from build123d import *

# Parameters (mm, degrees)
CYLINDER1393_R     = 1.7
CYLINDER1393_DEPTH = 8.5
CYLINDER1391_R     = 3.5
CYLINDER1391_DEPTH = 8.5


with BuildPart() as cylinder1393:
    # Cylinder1393 → Cylinder1393 (new body)
    with BuildSketch(Plane(origin=(436, 67, 100), x_dir=(0, 0, -1), z_dir=(1, 0, 0))):
        Circle(CYLINDER1393_R)
    extrude(amount=CYLINDER1393_DEPTH)


with BuildPart() as bucket_right_half_long_spacer:
    # Cylinder1391 → Cylinder1391 (new body)
    with BuildSketch(Plane(origin=(436, 67, 100), x_dir=(0, 0, -1), z_dir=(1, 0, 0))):
        Circle(CYLINDER1391_R)
    extrude(amount=CYLINDER1391_DEPTH)

    # Cut014358: cut Cylinder1393
    add(cylinder1393.part, mode=Mode.SUBTRACT)


with BuildPart() as bucket_right_half_long_spacer_1:
    # Cut014358 placement: moved
    add(bucket_right_half_long_spacer.part.moved(Location((42, 0, 0))))


solid = bucket_right_half_long_spacer_1.part
Work out the finished part from the listing and answer in its coordinate system (mm). Coordinates: 2 decimals unless noted, no trailing zeros. Loops run counter-clockwise (first coordinate to the right, second up) from the corner with the lowest first, then second, coordinate; pieces in that order, holes last. Notation, with made-up numbers: M 70.25,-16 L 98.25,-16 A22 cw 98.25,7 Z; hole C 47,30 d5. An arc over 180 degrees is marked long. Answer in a Markdown table with one row per item. Add a question column.
1. The mould has two halves that part along Z. Classify faces 1 (the flat face through (478, 68, 98)), 2 (the cylindrical face through (482.19, 67.07, 101.7)), 3 (the cylindrical face through (482.19, 65.659, 96.767)): pulls with the +Z half, pulls with the -Z half, needs draft (parallel to the pull), parting line crosses it, or undercut.
2. Find section B-B, the plane y = 67. Write down the section's boundary in (x, z), then the cut area to 3 significant figures.
3. Consider L1, parallel to Y at x = 482.75, z = 100; L2, parallel to Y at x = 480.25, z = 98.75; L3, parallel to Z at x = 479, y = 68.25. Determine where each line is inside the solid, lowest interval first.
4. Flat-ended cylindrical pins translate along their axes: P1, Ø2, axis at x = 482.5, y = 68, coming from the -Z side; P2, Ø3, axis at y = 67, z = 100, coming from the -X side. Find the tip coordinate at first contact, or state that the pin passes through.
5. Find section A-A, the plane z = 100. Write down the section's boundary in (x, y), then the cut area to 3 significant figures.
6. Find section C-C, the plane x = 484.5. Write down the section's boundary in (y, z).
7. Find section D-D, the plane y = 64. Write down the section's boundary in (x, z), then the cut area to 3 significant figures.
Reported:
| question | item | result |
|---|---|---|
| 1 | face 1 | needs draft |
| 1 | face 2 | undercut |
| 1 | face 3 | parting line crosses it |
| 2 | outline | M 478,96.5 L 486.5,96.5 L 486.5,98.3 L 478,98.3 Z; M 478,101.7 L 486.5,101.7 L 486.5,103.5 L 478,103.5 Z |
| 2 | area | 30.6 mm^2 |
| 3 | L1 | y = 63.5 to 65.3, 68.7 to 70.5 |
| 3 | L2 | y = 63.73 to 65.85, 68.15 to 70.27 |
| 3 | L3 | z = 96.73 to 98.85, 101.15 to 103.27 |
| 4 | P1 | stops at z = 96.5 |
| 4 | P2 | passes through |
| 5 | outline | M 478,63.5 L 486.5,63.5 L 486.5,65.3 L 478,65.3 Z; M 478,68.7 L 486.5,68.7 L 486.5,70.5 L 478,70.5 Z |
| 5 | area | 30.6 mm^2 |
| 6 | outline | C 67,100 d7; hole C 67,100 d3.4 |
| 7 | outline | M 478,98.2 L 486.5,98.2 L 486.5,101.8 L 478,101.8 Z |
| 7 | area | 30.6 mm^2 |
